Model file for the job. Use its own axes, mm. A direction names the side the tool comes from. Round coordinates to 2 decimals unless told otherwise and drop trailing zeros. Write each loop counter-clockwise with the first axis right and the second up, starting at its lowest first coordinate (ties: lowest second). Pieces come first, ordered by that corner, then holes. Notation, with made-up numbers: (48.5, 23) - (86.5, 23) arc R16 ccw to (86.5, 27) - close; hole circle Ø4 at (35.5, 22.5). An arc over 180 degrees is marked (long way). One line per item, written item: value.
from build123d import *

# Parameters (mm, degrees)
SKETCH_1_W                = 38
SKETCH_1_H                = 11.4
EXTRUDE_1_DEPTH           = 1.6
SKETCH_1_4_W              = 4
SKETCH_1_4_H              = 14
EXTRUDE_2_DEPTH           = 5
SKETCH_2_W                = 0.1
SKETCH_2_H                = 1.3
SKETCH_2_W_2              = 10
SKETCH_2_W_3              = 2
CUT_EXTRUDE_1_DEPTH       = 21.856653615
CUT_EXTRUDE_START         = 7
CUT_EXTRUDE_2_DEPTH       = 2.1
CUT_EXTRUDE_START_2       = -4.9
CUT_EXTRUDE_3_DEPTH       = 2.1
CUT_EXTRUDE_6_DEPTH       = 21.856653615
CUT_EXTRUDE_6_DEPTH_BACK  = 21.856653615
EXTRUDE_START             = 5.1
SKETCH_4_6_R              = 2.25
EXTRUDE_3_DEPTH           = 1.9
EXTRUDE_START_2           = -7
SKETCH_4_7_R              = 2.25
EXTRUDE_4_DEPTH           = 1.9
CUT_EXTRUDE_7_DEPTH       = 22.386970332
CUT_EXTRUDE_7_DEPTH_BACK  = 22.386970332
SKETCH_3_R                = 0.65
SKETCH_3_R_2              = 0.55
CUT_EXTRUDE_START_3       = 3
CUT_EXTRUDE_8_DEPTH       = 2.1
CUT_EXTRUDE_START_4       = -5.1
SKETCH_5_2_R              = 2.5
SKETCH_5_2_W              = 2.5
SKETCH_5_2_H              = 2.5
CUT_EXTRUDE_9_DEPTH       = 5.1
CUT_EXTRUDE_10_DEPTH      = 22.386970332
CUT_EXTRUDE_10_DEPTH_BACK = 22.386970332
EXTRUDE_START_3           = 3
EXTRUDE_5_DEPTH           = 1.9
EXTRUDE_START_4           = -4.9
EXTRUDE_6_DEPTH           = 1.9
CUT_EXTRUDE_11_DEPTH      = 22.386970332
CUT_EXTRUDE_11_DEPTH_BACK = 22.386970332
SKETCH_3_3_R              = 0.65
SKETCH_3_3_R_2            = 0.55
CUT_EXTRUDE_12_DEPTH      = 22.386970332
CUT_EXTRUDE_12_DEPTH_BACK = 22.386970332
SKETCH_9_W                = 15.45
SKETCH_9_H                = 0.397025916
SKETCH_10_W               = 38
SKETCH_10_H               = 1.5
EXTRUDE_7_DEPTH           = 1.5
FILLET_1_R                = 1
SKETCH_11_W               = 4.7
SKETCH_11_H               = 4.602974084
CUT_EXTRUDE_13_DEPTH      = 17.397649411
CUT_EXTRUDE_START_5       = 4.9
SKETCH_11_2_W             = 4.7
SKETCH_11_2_H             = 4.602974084
CUT_EXTRUDE_14_DEPTH      = 17.397649411
CUT_EXTRUDE_START_6       = 5.1
SKETCH_11_4_W             = 4.7
SKETCH_11_4_H             = 4.602974084
CUT_EXTRUDE_15_DEPTH      = 10.2


# Read off the part's stored shape, not the designer's step: 切除-拉伸8, 凸台-拉伸5, 凸台-拉伸6
with BuildPart() as part:
    # 草图1 → 凸台-拉伸1 (new body)
    with BuildSketch(Plane(origin=(0, 0, 0), x_dir=(1, 0, 0), z_dir=(0, 1, 0))):
        Rectangle(SKETCH_1_W, SKETCH_1_H)
    extrude(amount=EXTRUDE_1_DEPTH)

    # 草图1<4> → 凸台-拉伸2 (add)
    with BuildSketch(Plane(origin=(0, 0, 0), x_dir=(1, 0, 0), z_dir=(0, 1, 0))):
        with Locations((-5, 0)):
            Rectangle(SKETCH_1_4_W, SKETCH_1_4_H)
        with Locations((5, 0)):
            Rectangle(SKETCH_1_4_W, SKETCH_1_4_H)
    extrude(amount=-EXTRUDE_2_DEPTH)

    # 草图2 → 切除-拉伸1 (cut, through all)
    with BuildSketch(Plane(origin=(0, 0, 0), x_dir=(1, 0, 0), z_dir=(0, 1, 0))):
        with Locations((-5.05, 6.35)):
            Rectangle(SKETCH_2_W, SKETCH_2_H)
        with Locations((0, 6.35)):
            Rectangle(SKETCH_2_W_2, SKETCH_2_H)
        with Locations((5.05, 6.35)):
            Rectangle(SKETCH_2_W, SKETCH_2_H)
        with Locations((-6, -6.35)):
            Rectangle(SKETCH_2_W_3, SKETCH_2_H)
        with Locations((-4.95, -6.35)):
            Rectangle(SKETCH_2_W, SKETCH_2_H)
        with Locations((4.95, -6.35)):
            Rectangle(SKETCH_2_W, SKETCH_2_H)
        with Locations((6, -6.35)):
            Rectangle(SKETCH_2_W_3, SKETCH_2_H)
    extrude(amount=-CUT_EXTRUDE_1_DEPTH, mode=Mode.SUBTRACT)

    # 草图4 → 切除-拉伸2 (cut)
    with BuildSketch(Plane(origin=(0, 0, 0), x_dir=(0, 0, -1), z_dir=(1, 0, 0)).offset(CUT_EXTRUDE_START)):
        with BuildLine():
            ThreePointArc((-3.7, -2.5), (-4.263508327, -0.91886117), (-5.7, -0.050510257))
            Line((-5.7, -0.050510257), (-5.7, -5))
            Line((-5.7, -5), (-3.7, -5))
            Line((-3.7, -5), (-3.7, -2.5))
        make_face()
    extrude(amount=-CUT_EXTRUDE_2_DEPTH, mode=Mode.SUBTRACT)

    # 草图4<3> → 切除-拉伸3 (cut)
    with BuildSketch(Plane(origin=(0, 0, 0), x_dir=(0, 0, -1), z_dir=(1, 0, 0)).offset(CUT_EXTRUDE_START_2)):
        with BuildLine():
            ThreePointArc((-3.7, -2.5), (-4.263508327, -0.91886117), (-5.7, -0.050510257))
            Line((-5.7, -0.050510257), (-5.7, -5))
            Line((-5.7, -5), (-3.7, -5))
            Line((-3.7, -5), (-3.7, -2.5))
        make_face()
    extrude(amount=-CUT_EXTRUDE_3_DEPTH, mode=Mode.SUBTRACT)

    # 草图4<5> → 切除-拉伸6 (cut, two sides: drawn at the far end of the back side and taken through both)
    with BuildSketch(Plane(origin=(0, 0, 0), x_dir=(0, 0, -1), z_dir=(1, 0, 0)).offset(-CUT_EXTRUDE_6_DEPTH_BACK)):
        with BuildLine():
            Line((8.45, 0), (5.7, 0))
            Line((5.7, 0), (5.7, -0.306258903))
            ThreePointArc((5.7, -0.306258903), (7.60312152, -0.74109409), (8.45, -2.5))
            Line((8.45, -2.5), (8.45, 0))
        make_face()
        with BuildLine():
            Line((8.45, -5), (8.45, -2.5))
            ThreePointArc((8.45, -2.5), (7.60312152, -4.25890591), (5.7, -4.693741097))
            Line((5.7, -4.693741097), (5.7, -5))
            Line((5.7, -5), (8.45, -5))
        make_face()
    extrude(amount=CUT_EXTRUDE_6_DEPTH + CUT_EXTRUDE_6_DEPTH_BACK, mode=Mode.SUBTRACT)

    # 草图4<6> → 凸台-拉伸3 (add)
    with BuildSketch(Plane(origin=(0, 0, 0), x_dir=(0, 0, -1), z_dir=(1, 0, 0)).offset(EXTRUDE_START)):
        with Locations((6.2, -2.5)):
            Circle(SKETCH_4_6_R)
    extrude(amount=EXTRUDE_3_DEPTH)

    # 草图4<7> → 凸台-拉伸4 (add)
    with BuildSketch(Plane(origin=(0, 0, 0), x_dir=(0, 0, -1), z_dir=(1, 0, 0)).offset(EXTRUDE_START_2)):
        with Locations((6.2, -2.5)):
            Circle(SKETCH_4_7_R)
    extrude(amount=EXTRUDE_4_DEPTH)

    # 草图3 → 切除-拉伸7 (cut, two sides: drawn at the far end of the back side and taken through both)
    with BuildSketch(Plane(origin=(0, 0, 0), x_dir=(0, 0, -1), z_dir=(1, 0, 0)).offset(-CUT_EXTRUDE_7_DEPTH_BACK)):
        with Locations(Location((-6.2, -2.5, 0), (0, 0, 180))):
            Circle(SKETCH_3_R)
        with Locations(Location((6.2, -2.5, 0), (0, 0, 204.619977329))):
            Circle(SKETCH_3_R_2)
    extrude(amount=CUT_EXTRUDE_7_DEPTH + CUT_EXTRUDE_7_DEPTH_BACK, mode=Mode.SUBTRACT)

    # 切除-拉伸8 outline → 切除-拉伸8 (cut)
    with BuildSketch(Plane(origin=(0, 0, 0), x_dir=(0, 0, -1), z_dir=(1, 0, 0)).offset(CUT_EXTRUDE_START_3)):
        with BuildLine():
            Line((3.7, -2.5), (3.7, -5))
            Line((3.7, -5), (5.7, -5))
            Line((5.7, -5), (5.7, -2.729128785))
            ThreePointArc((5.7, -2.729128785), (5.65, -2.5), (5.7, -2.270871215))
            Line((5.7, -2.270871215), (5.7, -0.050510257))
            ThreePointArc((5.7, -0.050510257), (4.263508327, -0.91886117), (3.7, -2.5))
        make_face()
    extrude(amount=CUT_EXTRUDE_8_DEPTH, mode=Mode.SUBTRACT)

    # 草图5<2> → 切除-拉伸9 (cut)
    with BuildSketch(Plane(origin=(0, 0, 0), x_dir=(0, 0, -1), z_dir=(1, 0, 0)).offset(CUT_EXTRUDE_START_4)):
        with Locations((6.2, -2.5)):
            Circle(SKETCH_5_2_R)
        with Locations((4.95, -3.75)):
            Rectangle(SKETCH_5_2_W, SKETCH_5_2_H)
    extrude(amount=CUT_EXTRUDE_9_DEPTH, mode=Mode.SUBTRACT)

    # 草图7 → 切除-拉伸10 (cut, two sides: drawn at the far end of the back side and taken through both)
    with BuildSketch(Plane(origin=(0, 0, 0), x_dir=(0, 0, -1), z_dir=(1, 0, 0)).offset(-CUT_EXTRUDE_10_DEPTH_BACK)):
        with BuildLine():
            Line((-5.7, -0.306258903), (-5.7, 0))
            Line((-5.7, 0), (-8.45, 0))
            Line((-8.45, 0), (-8.45, -2.5))
            ThreePointArc((-8.45, -2.5), (-7.60312152, -0.74109409), (-5.7, -0.306258903))
        make_face()
    extrude(amount=CUT_EXTRUDE_10_DEPTH + CUT_EXTRUDE_10_DEPTH_BACK, mode=Mode.SUBTRACT)

    # 凸台-拉伸5 outline → 凸台-拉伸5 (add)
    with BuildSketch(Plane(origin=(0, 0, 0), x_dir=(0, 0, -1), z_dir=(1, 0, 0)).offset(EXTRUDE_START_3)):
        with BuildLine():
            Line((-7, -4.602974084), (-7, -0.397025915))
            ThreePointArc((-7, -0.397025915), (-8.45, -2.5), (-7, -4.602974084))
        make_face()
        with BuildLine():
            ThreePointArc((-5.7, -2.084668807), (-6.85, -2.5), (-5.7, -2.915331193))
            Line((-5.7, -2.915331193), (-5.7, -2.084668807))
        make_face()
    extrude(amount=EXTRUDE_5_DEPTH)

    # 凸台-拉伸6 outline → 凸台-拉伸6 (add)
    with BuildSketch(Plane(origin=(0, 0, 0), x_dir=(0, 0, -1), z_dir=(1, 0, 0)).offset(EXTRUDE_START_4)):
        with BuildLine():
            Line((-7, -4.602974084), (-7, -0.397025915))
            ThreePointArc((-7, -0.397025915), (-8.45, -2.5), (-7, -4.602974084))
        make_face()
        with BuildLine():
            ThreePointArc((-5.7, -2.084668807), (-6.85, -2.5), (-5.7, -2.915331193))
            Line((-5.7, -2.915331193), (-5.7, -2.084668807))
        make_face()
    extrude(amount=EXTRUDE_6_DEPTH)

    # 草图3<3> → 切除-拉伸11 (cut, two sides: drawn at the far end of the back side and taken through both)
    with BuildSketch(Plane(origin=(0, 0, 0), x_dir=(0, 0, -1), z_dir=(1, 0, 0)).offset(-CUT_EXTRUDE_11_DEPTH_BACK)):
        with Locations(Location((-6.2, -2.5, 0), (0, 0, 180))):
            Circle(SKETCH_3_3_R)
        with Locations(Location((6.2, -2.5, 0), (0, 0, 180))):
            Circle(SKETCH_3_3_R_2)
    extrude(amount=CUT_EXTRUDE_11_DEPTH + CUT_EXTRUDE_11_DEPTH_BACK, mode=Mode.SUBTRACT)

    # 草图9 → 切除-拉伸12 (cut, two sides: drawn at the far end of the back side and taken through both)
    with BuildSketch(Plane(origin=(0, 0, 0), x_dir=(0, 0, -1), z_dir=(1, 0, 0)).offset(-CUT_EXTRUDE_12_DEPTH_BACK)):
        with Locations((0.725, -4.801487042)):
            Rectangle(SKETCH_9_W, SKETCH_9_H)
    extrude(amount=CUT_EXTRUDE_12_DEPTH + CUT_EXTRUDE_12_DEPTH_BACK, mode=Mode.SUBTRACT)

    # 草图10 → 凸台-拉伸7 (add)
    with BuildSketch(Plane(origin=(0, 1.6, 0), x_dir=(1, 0, 0), z_dir=(0, 1, 0))):
        with Locations((0, 3.45)):
            Rectangle(SKETCH_10_W, SKETCH_10_H)
        with Locations((0, -3.45)):
            Rectangle(SKETCH_10_W, SKETCH_10_H)
    extrude(amount=EXTRUDE_7_DEPTH)

    # 圆角1
    fillet_1_edges = [part.edges().sort_by_distance(p)[0] for p in [
        (5.95, -4.602974084, 3.7),
        (4.05, -4.602974084, -3.7),
        (-4.05, -4.602974084, -3.7),
        (-5.95, -4.602974084, 3.7),
    ]]
    fillet(fillet_1_edges, radius=FILLET_1_R)

    # 草图11 → 切除-拉伸13 (cut, through all)
    with BuildSketch(Plane(origin=(0, 0, 0), x_dir=(0, 0, -1), z_dir=(1, 0, 0)).offset(CUT_EXTRUDE_START_2)):
        with Locations((-3.35, -2.301487042)):
            Rectangle(SKETCH_11_W, SKETCH_11_H)
    extrude(amount=-CUT_EXTRUDE_13_DEPTH, mode=Mode.SUBTRACT)

    # 草图11<2> → 切除-拉伸14 (cut, through all)
    with BuildSketch(Plane(origin=(0, 0, 0), x_dir=(0, 0, -1), z_dir=(1, 0, 0)).offset(CUT_EXTRUDE_START_5)):
        with Locations((-3.35, -2.301487042)):
            Rectangle(SKETCH_11_2_W, SKETCH_11_2_H)
    extrude(amount=CUT_EXTRUDE_14_DEPTH, mode=Mode.SUBTRACT)

    # 草图11<4> → 切除-拉伸15 (cut)
    with BuildSketch(Plane(origin=(0, 0, 0), x_dir=(0, 0, -1), z_dir=(1, 0, 0)).offset(CUT_EXTRUDE_START_6)):
        with Locations((3.35, -2.301487042)):
            Rectangle(SKETCH_11_4_W, SKETCH_11_4_H)
    extrude(amount=-CUT_EXTRUDE_15_DEPTH, mode=Mode.SUBTRACT)


solid = part.part
1. Band-saw the part on B-B on y = 2.5. Write the cut outline in (x, z), plus the area to 3 significant figures.
Report:
outline: (-19, -4.2) - (19, -4.2) - (19, -2.7) - (-19, -2.7) - close; (-19, 2.7) - (19, 2.7) - (19, 4.2) - (-19, 4.2) - close
area: 114 mm²
2. Tool access for faces 4 (the face through (0, 2, 2.7)), 5 (the face through (5.1, -2, -5)), 6 (the face through (0, 1.6, 5)), 7 (the face through (-4.9, -2, 5)), 8 (the face through (0, 2, -4.2)): list every direction of +Z, -Z, +X, -X, +Y, -Y with a clear straight run to the whole face (end or side of a thin tool).
Report:
face 4: +X, -X, +Y
face 5: -Z, -Y
face 6: +Z, +X, -X, +Y
face 7: +Z, -X, -Y
face 8: -Z, +X, -X, +Y
3. Band-saw the part on C-C on x = 0.5. Write the cut outline in (y, z), plus the area to 3 significant figures.
Report:
outline: (0, -5.7) - (1.6, -5.7) - (1.6, -4.2) - (3.1, -4.2) - (3.1, -2.7) - (1.6, -2.7) - (1.6, 2.7) - (3.1, 2.7) - (3.1, 4.2) - (1.6, 4.2) - (1.6, 5.7) - (0, 5.7) - close
area: 22.7 mm²
4. Mould opens along Y. For faces 1 (the face through (-5, -4.603, 0)), 2 (the face through (3.937, -1.865, 6.059)), 3 (the face through (-7, -2, -4)) say: released by +Y, released by -Y, zero draft, split by the parting line, or undercut.
Report:
face 1: released by -Y
face 2: undercut
face 3: zero draft
5. Drop flat-ended pins along their axis: pin 1 (1 mm diameter, centred on y = -2.5, z = 6.2, fed in from +X); pin 2 (1.6 mm diameter, centred on x = 8, y = 2, fed in from +Z); pin 3 (2 mm diameter, centred on x = -12, z = -1.5, fed in from +Y); pin 4 (3.5 mm diameter, centred on y = -2.5, z = -3.5, fed in from +X). Give the stop position or say it passes through.
Report:
pin 1: through
pin 2: z = 5.7
pin 3: y = 1.6
pin 4: x = 7
6. Wall check: probe 1 along Y at (x, z) = (-6.45, -6.2); probe 2 along Z at (x, y) = (5.5, -2.5); probe 3 along Z at (x, y) = (-4.25, -2.5). Give the ranges that are in metal, low to high. Write a range as [from, to].
Report:
probe 1: [-4.6, -3.05], [-1.95, -0.25]
probe 2: [-8.45, -6.75], [-5.65, 1]
probe 3: [-1, 5.55], [6.85, 8.45]
7. Band-saw the part on D-D on z = -3.25. Write the cut outline in (x, y), plus the area to 3 significant figures.
Report:
outline: (-19, 0) - (-7, 0) - (-7, -4.6) - (-5.1, -4.6) - (-5.1, 0) - (5.1, 0) - (5.1, -4.6) - (7, -4.6) - (7, 0) - (19, 0) - (19, 3.1) - (-19, 3.1) - close
area: 135 mm²
8. Band-saw the part on A-A on z = -6.2. Write the cut outline in (x, y), plus the area to 3 significant figures.
Report:
outline: (-7, -4.6) - (-5.1, -4.6) - (-5.1, -3.05) - (-7, -3.05) - close; (-7, -1.95) - (-5.1, -1.95) - (-5.1, -0.25) - (-7, -0.25) - close; (5.1, -4.6) - (7, -4.6) - (7, -3.05) - (5.1, -3.05) - close; (5.1, -1.95) - (7, -1.95) - (7, -0.25) - (5.1, -0.25) - close
area: 12.4 mm²
